Build history of the part. All positions in model axes, mm. A direction names the side the tool comes from. Round coordinates to 2 decimals unless told otherwise and drop trailing zeros. Write each loop counter-clockwise with the first axis right and the second up, starting at its lowest first coordinate (ties: lowest second). Pieces come first, ordered by that corner, then holes. Notation, with made-up numbers: (82.5, -28) -> (138.5, -28) arc R24 ccw to (138.5, -15) -> close; hole circle Ø4 at (84.25, -26). An arc over 180 degrees is marked (long way). Return JSON: item names as keys, results as strings.
Autodesk Inventor part; units mm, degrees
ref_plane "Plano de trabajo1" through (64.5, -49.5, 12.8) normal (0, 0, 1) x (1, 0, 0)
ref_plane "YZ Plane" through (0, 0, 0) normal (1, 0, 0) x (0, 1, 0)
ref_plane "XZ Plane" through (0, 0, 0) normal (0, 1, 0) x (-1, 0, 0)
ref_plane "Plano de trabajo1" through (64.5, -49.5, 12.8) normal (0, 0, 1) x (1, 0, 0)
sketch "Boceto1" plane through (0, 0, 0) normal (0, 0, 1) x (1, 0, 0)
  line L0 (-63.5, 34.5) -> (63.5, 34.5)
  line L1 (63.5, -34.5) -> (-63.5, -34.5)
  line L2 (63.5, 34.5) -> (63.5, -34.5)
  line L3 (64.5, -16.5586) -> (64.5, -23.5586)
  line L4 (64.5, -23.5586) -> (64.5, -44.5)
  line L5 (64.5, -49.5) -> (64.5, -23.5586)
  line L6 (64.5, -16.5586) -> (64.5, -23.5586)
  line L7 (63.5, -34.5) -> (57.5, -34.5)
  line L8 (57.5, -34.5) -> (57.5, -9.5)
  line L9 (57.5, -9.5) -> (63.5, -9.5)
  line L10 (63.5, -9.5) -> (63.5, -34.5)
  point P0 (0, 0)
extrude "Extrusión1" add sketch "Boceto1" along normal up to surface (12.8 mm away)
sketch "Boceto2" plane through (57.5, -34.5, 0) normal (-1, 0, 0) x (0, 0, 1)
  line L0 (0, 0) -> (3, 0)
  line L1 (0, 25) -> (3, 25)
  line L2 (0, 25) -> (12.8, 25)
  line L3 (12.8, 0) -> (12.8, 25)
  arc A0 (12.8, 10.9414) -> (-1.2, 10.9414) centre (5.8, 10.9414) ccw
  arc A1 (12.8, 18.0828) -> (3, 20.5414) centre (5.8, 10.9414) ccw
  line L4 (3, 25) -> (3, 20.5414)
  line L5 (12.8, 0) -> (12.8, 5)
  line L6 (3, 1.3414) -> (3, 0)
  line L7 (3, 0) -> (12.8, 0)
  arc A2 (3, 1.3414) -> (12.8, 3.8) centre (5.8, 10.9414) ccw
  point P0 (0, 34.5)
  dimension "d4" = 3
  dimension "d6" = 3
  dimension "d8" = 3
  dimension "d9" = 5
extrude "Extrusión2" cut sketch "Boceto2" against normal up to surface (6 mm away)
hole "Agujero1" at (57.5, -23.5586, 5.8) direction (1, 0, 0) diameter 9 end up to surface
sketch "Boceto3" plane through (57.5, -34.5, 3) normal (0, 0, 1) x (1, 0, 0)
  line L0 (0, 5) -> (6, 5)
  line L1 (6, 0) -> (0, 0)
  line L2 (6, 25) -> (6, 20.5414)
  line L3 (0, 25) -> (6, 25)
  line L4 (0, 20.5414) -> (0, 25)
  line L5 (0, 20.5414) -> (6, 20.5414)
  line L6 (6, 5) -> (0, 0)
  line L7 (0, 20.5414) -> (6, 25)
  point P0 (-57.5, 34.5)
  point P1 (3, 22.7707)
  point P2 (3, 2.5)
hole "Agujero2" at (60.5, -11.7293, 3) at (60.5, -32, 3) direction (0, 0, -1) diameter 2.5 end up to surface
sketch "Boceto4" plane through (57.5, -16.4172, 12.8) normal (0, 0, 1) x (1, 0, 0)
  arc A0 (2.5308, -16.7414) -> (3.4692, -16.7414) centre (3, -15.5828) ccw
  circle A1 centre (3, -15.5828) radius 2
  point P0 (-57.5, 16.4172)
  dimension "d30" = 4
extrude "Extrusión3" cut sketch "Boceto4" against normal up to surface (9.8 mm away)
properties part number "soporteDerecho"
Q1. Saw through at D-D on y = -23.25. List the corners of the cut face in (x, z), then the cut area to 3 significant figures.
Verdict:
{"outline": "(57.5, 0) -> (63.5, 0) -> (63.5, 1.31) -> (57.5, 1.31) -> close; (57.5, 10.29) -> (63.5, 10.29) -> (63.5, 12.8) -> (57.5, 12.8) -> close", "area": "22.9 mm²"}
Q2. Wall check: L1, parallel to Y at x = 63, z = 6; L2, parallel to Y at x = 60, z = 2.75; L3, parallel to X at y = -32, z = 0.8. Give the ranges that are in metal, low to high.
Verdict:
{"L1": "y = -33.56 to -28.05, -19.06 to -13.56", "L2": "y = -34.5 to -33.15, -30.85 to -26.87, -20.25 to -12.87, -10.58 to -9.5", "L3": "x = 57.5 to 59.25, 61.75 to 63.5"}
Q3. Pin check, flat tips, straight feed: pin 1 Ø3 at (x, z) = (58.5, 7.5) entering from +Y; pin 2 Ø1 at (x, z) = (61, 10.5) entering from -Y; pin 3 Ø3 at (x, y) = (60.5, -32) entering from +Z. Stop position of each tip, or through.
Verdict:
{"pin 1": "stops at y = -13.56", "pin 2": "stops at y = -30.27", "pin 3": "stops at z = 3"}
Q4. Saw through at A-A on x = 60.5. List the corners of the cut face in (y, z).
Verdict:
{"outline": "(-34.5, 0) -> (-33.25, 0) -> (-33.25, 3) -> (-34.5, 3) -> close; (-30.75, 0) -> (-12.98, 0) -> (-12.98, 3) -> (-13.96, 3) arc R10 ccw to (-16.42, 12.8) -> (-30, 12.8) -> (-30, 3) -> (-30.75, 3) -> close; (-10.48, 0) -> (-9.5, 0) -> (-9.5, 3) -> (-10.48, 3) -> close; hole circle Ø9 at (-23.56, 5.8)"}
Q5. Saw through at C-C on y = -32. List the corners of the cut face in (x, z), then the cut area to 3 significant figures.
Verdict:
{"outline": "(57.5, 0) -> (59.25, 0) -> (59.25, 3) -> (58.5, 3) -> (58.5, 11.16) -> (57.5, 11.16) -> close; (61.75, 0) -> (63.5, 0) -> (63.5, 11.16) -> (62.5, 11.16) -> (62.5, 3) -> (61.75, 3) -> close", "area": "26.8 mm²"}
Q6. 3-axis set-ups, long thin cutter, end or side, ignore diameter. For faces 1 (the cylindrical face through (60.542, -19.166, 4.824)), 2 (the flat face through (59, -12, 3)): which of +Z, -Z, +X, -X, +Y, -Y reach the whole face in a straight line?
Verdict:
{"face 1": "+X, -X", "face 2": "+X, -X, +Y"}
Q7. Saw through at B-B on z = 5.8. List the corners of the cut face in (x, y).
Verdict:
{"outline": "(57.5, -33.56) -> (59.25, -33.56) arc R2 cw (long way) to (61.75, -33.56) -> (63.5, -33.56) -> (63.5, -28.06) -> (57.5, -28.06) -> close; (57.5, -19.06) -> (63.5, -19.06) -> (63.5, -13.56) -> (57.5, -13.56) -> close"}
Q8. Two-plate mould, pull along X, no slides. Class faces 3 (the cylindrical face through (60.57, -30, 6.88)), 4 (the flat face through (59.79, -33.22, 3)), 5 (the flat face through (60, -22, 0)), 6 (the flat face through (57.5, -19, 8)): +X half, -X half, draft (parallel to the pull), parting line (faces both ways), or undercut.
Verdict:
{"face 3": "undercut", "face 4": "undercut", "face 5": "draft", "face 6": "-X half"}
